from build123d import *

# Parameters (mm, degrees)
SKETCH1_W           = 50
SKETCH1_H           = 30
BOSS_EXTRUDE1_DEPTH = 30
SKETCH3_R           = 5.933342005
CUT_EXTRUDE1_DEPTH  = 40
SKETCH4_W           = 1.254965376
SKETCH4_H           = 1
CUT_EXTRUDE2_DEPTH  = 51


with BuildPart() as part:
    # Sketch1 → Boss-Extrude1 (new body)
    with BuildSketch(Plane(origin=(0, 0, 0), x_dir=(0, 0, -1), z_dir=(1, 0, 0))):
        Rectangle(SKETCH1_W, SKETCH1_H)
    extrude(amount=BOSS_EXTRUDE1_DEPTH)

    # Sketch3 → Cut-Extrude1 (cut)
    with BuildSketch(Plane(origin=(0, 0, -25), x_dir=(-1, 0, 0), z_dir=(0, 0, -1))):
        with Locations((-15, 0)):
            Circle(SKETCH3_R)
    extrude(amount=-CUT_EXTRUDE1_DEPTH, mode=Mode.SUBTRACT)

    # Sketch4 → Cut-Extrude2 (cut, through all)
    with BuildSketch(Plane(origin=(0, 0, -25), x_dir=(-1, 0, 0), z_dir=(0, 0, -1))):
        with Locations((-29.372517312, 6.5)):
            Rectangle(SKETCH4_W, SKETCH4_H)
        with Locations((-29.372517312, -6.5)):
            Rectangle(SKETCH4_W, SKETCH4_H)
        with Locations((-0.627482688, -6.5)):
            Rectangle(SKETCH4_W, SKETCH4_H)
        with Locations((-0.627482688, 6.5)):
            Rectangle(SKETCH4_W, SKETCH4_H)
    extrude(amount=-CUT_EXTRUDE2_DEPTH, mode=Mode.SUBTRACT)


solid = part.part
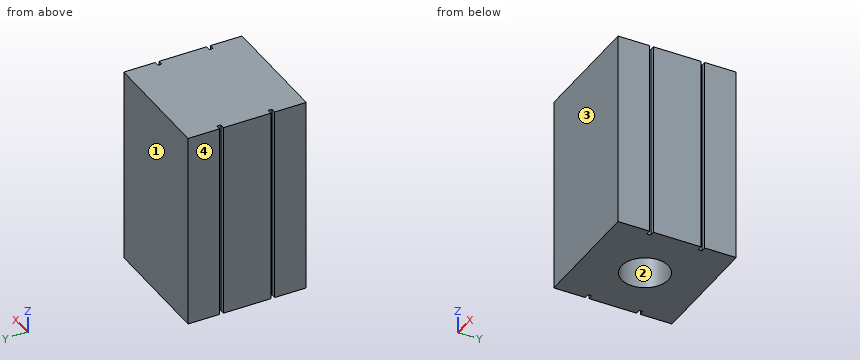
Read the model definition and answer for the solid it produces. Units are mm, in the model's axes. Face numbers are marked on the shaded views. Round coordinates to 2 decimals unless told otherwise and drop trailing zeros. Write each loop counter-clockwise with the first axis right and the second up, starting at its lowest first coordinate (ties: lowest second). Pieces come first, ordered by that corner, then holes. Notation, with made-up numbers: (11, 86.5) - (60, 86.5) arc R12 ccw to (60, 106.5) - close; hole circle Ø4 at (80.5, 9.5). An arc over 180 degrees is marked (long way). Use a Markdown table: item, result.
(1) The mould has two halves that part along Y. Classify the marked faces 1, 2, 3 and 4: released by +Y, released by -Y, zero draft, split by the parting line, or undercut.
Reported:
| item | result |
|---|---|
| face 1 | released by +Y |
| face 2 | undercut |
| face 3 | released by -Y |
| face 4 | zero draft |
(2) The part is cut by section C-C (x = 15). Write down the section's boundary in (y, z).
Reported:
| item | result |
|---|---|
| outline | (-15, -25) - (-5.93, -25) - (-5.93, 15) - (5.93, 15) - (5.93, -25) - (15, -25) - (15, 25) - (-15, 25) - close |
(3) The part is cut by section A-A (z = -2). Write down the section's boundary in (x, y), then the cut area to 3 significant figures.
Reported:
| item | result |
|---|---|
| outline | (0, -15) - (30, -15) - (30, -7) - (28.75, -7) - (28.75, -6) - (30, -6) - (30, 6) - (28.75, 6) - (28.75, 7) - (30, 7) - (30, 15) - (0, 15) - (0, 7) - (1.25, 7) - (1.25, 6) - (0, 6) - (0, -6) - (1.25, -6) - (1.25, -7) - (0, -7) - close; hole circle Ø11.87 at (15, 0) |
| area | 784 mm2 |
(4) Straight lines are drawn through the part: line 1 along Y through (x, z) = (15, -4); line 2 along Z through (x, y) = (13.75, -1.5); line 3 along X through (y, z) = (2.25, 12). For each, find the intervals that lie inside material, in ascending order. Write a range as [from, to].
Reported:
| item | result |
|---|---|
| line 1 | [-15, -5.93], [5.93, 15] |
| line 2 | [15, 25] |
| line 3 | [0, 9.51], [20.49, 30] |
(5) The part is cut by section B-B (y = 0). Write down the section's boundary in (x, z), then the cut area to 3 significant figures.
Reported:
| item | result |
|---|---|
| outline | (0, -25) - (9.07, -25) - (9.07, 15) - (20.93, 15) - (20.93, -25) - (30, -25) - (30, 25) - (0, 25) - close |
| area | 1,030 mm2 |
(6) Each of these flat-tipped pins is pushed along its axis until it touches: pin 1 Ø6 at (x, y) = (16.5, 1.5) entering from -Z; pin 2 Ø0.8 at (y, z) = (-6.5, -6) entering from +X. Where does it stop, or does it pass through?
Reported:
| item | result |
|---|---|
| pin 1 | z = 15 |
| pin 2 | x = 28.75 |
